```python
from build123d import *

# Parameters (mm, degrees)
F0_W      = 4.96
F0_H      = 15.83
F1_DEPTH  = 6.36
F2_R      = 2.45
F3_DEPTH  = 1.84
F4_R      = 2.45
F5_DEPTH  = 1.87
F6_R      = 2.45
F7_DEPTH  = 1.87
F9_D      = 3.14
F10_R     = 2.45
F11_DEPTH = 1.43
F12_R     = 2.45
F13_DEPTH = 1.43
F14_R     = 1.57
F15_DEPTH = 5.06
F16_R     = 1.57
F17_DEPTH = 1.43
F18_R     = 1.6
F19_DEPTH = 6.435
F20_R     = 1.7
F21_DEPTH = 1.41
F22_R     = 1.6
F23_DEPTH = 6.435
F24_R     = 1.7
F25_DEPTH = 1.41


with BuildPart() as f1:
    # F0 (on Front) → F1 (new body)
    with BuildSketch(Plane.XZ):
        with Locations((-27.94799, 11.446154)):
            Rectangle(F0_W, F0_H)
    extrude(amount=F1_DEPTH)

    # F2 (on face) → F3 (join)
    with BuildSketch(Plane.XZ.offset(6.36)):
        with Locations((-27.94799, 15.941154)):
            Circle(F2_R)
    extrude(amount=F3_DEPTH)

    # F4 (on face) → F5 (join)
    with BuildSketch(Plane.XY.offset(19.361154)):
        with Locations((-27.94799, -3.18)):
            Circle(F4_R)
    extrude(amount=F5_DEPTH)

    # F6 (on face) → F7 (join)
    with BuildSketch(Plane(origin=(0, 0, 3.531154), x_dir=(1, 0, 0), z_dir=(0, 0, -1))):
        with Locations((-27.94799, 3.18)):
            Circle(F6_R)
    extrude(amount=F7_DEPTH)

    # F9 (through all)
    with Locations(Plane(origin=(0, 0, 1.661154), x_dir=(1, 0, 0), z_dir=(0, 0, -1))):
        with Locations((-27.94799, 3.18)):
            Hole(F9_D / 2)

    # F10 (on face) → F11 (join)
    with BuildSketch(Plane.YZ.offset(-25.46799)):
        with Locations((-3.18, 15.941154)):
            Circle(F10_R)
    extrude(amount=F11_DEPTH)

    # F12 (on face) → F13 (join)
    with BuildSketch(Plane(origin=(-30.42799, 0, 0), x_dir=(0, -1, 0), z_dir=(-1, 0, 0))):
        with Locations((3.18, 15.941154)):
            Circle(F12_R)
    extrude(amount=F13_DEPTH)

    # F14 (on face) → F15 (join)
    with BuildSketch(Plane.XZ.offset(6.36)):
        with Locations((-27.94799, 6.951154)):
            Circle(F14_R)
    extrude(amount=F15_DEPTH)

    # F16 (on face) → F17 (join)
    with BuildSketch(Plane(origin=(0, 0, 0), x_dir=(-1, 0, 0), z_dir=(0, 1, 0))):
        with Locations((27.94799, 15.941154)):
            Circle(F16_R)
        with Locations((27.94799, 6.951154)):
            Circle(F16_R)
    extrude(amount=F17_DEPTH)

    # F18 (on face) → F19 (join)
    with BuildSketch(Plane(origin=(-31.85799, 0, 0), x_dir=(0, -1, 0), z_dir=(-1, 0, 0))):
        with Locations((3.18, 15.941154)):
            Circle(F18_R)
    extrude(amount=F19_DEPTH)

    # F20 (on face) → F21 (join)
    with BuildSketch(Plane(origin=(-38.29299, 0, 0), x_dir=(0, -1, 0), z_dir=(-1, 0, 0))):
        with Locations((3.18, 15.941154)):
            Circle(F20_R)
    extrude(amount=F21_DEPTH)

    # F22 (on face) → F23 (join)
    with BuildSketch(Plane.YZ.offset(-24.03799)):
        with Locations((-3.18, 15.941154)):
            Circle(F22_R)
    extrude(amount=F23_DEPTH)

    # F24 (on face) → F25 (join)
    with BuildSketch(Plane.YZ.offset(-17.60299)):
        with Locations((-3.18, 15.941154)):
            Circle(F24_R)
    extrude(amount=F25_DEPTH)


solid = f1.part
```
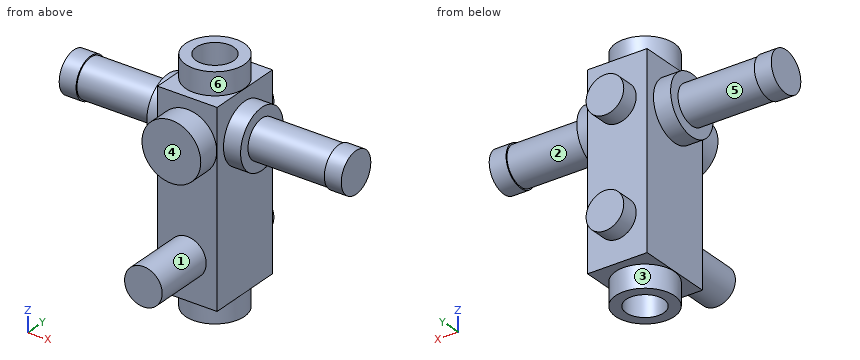
Geometry: final body of the model. Coordinates: model frame, mm. Face numbers are marked on the shaded views. A direction names the side the tool comes from. Round coordinates to 2 decimals unless told otherwise and drop trailing zeros. Write each loop counter-clockwise with the first axis right and the second up, starting at its lowest first coordinate (ties: lowest second). Pieces come first, ordered by that corner, then holes.
Item 1: Mould query, pull axis Z, two halves, no side actions, for the marked faces 1, 2 and 3. Classes: +Z half, -Z half, draft (parallel to the pull), parting line (faces both ways), or undercut.
Item 2: Set-up query: the marked faces 4, 5 and 6. Return all of +Z, -Z, +X, -X, +Y, -Y with unobstructed straight access to the full face (end or side cutting, diameter ignored); none if empty.
Item 3: Pin query (flat end, axial travel): P1, Ø1.5, axis at y = -8, z = 18, coming from the +X side; P2, Ø2, axis at x = -24, y = -1.5, coming from the +Z side; P3, Ø4, axis at x = -30.5, z = 15, coming from the -Y side. Return the tip coordinate at first contact, or that it passes through.
Item 4: Section query D-D (y = -10.25). Return loops of the section in (x, z).
Item 5: Section query A-A (z = 18.75). Return loops of the section in (x, y), plus the area to 3 significant figures.
Item 6: Material intervals for L1, parallel to X at y = -5.25, z = 8.5; L2, parallel to X at y = -4.5, z = 6.5; L3, parallel to Z at x = -35, y = -3.25, sorted ascending.
Item 7: Section query C-C (x = -20.75). Return loops of the section in (y, z), plus the area to 3 significant figures.
Completed:
1. face 1: undercut
1. face 2: parting line
1. face 3: draft
2. face 4: +Z, +X, -X, -Y
2. face 5: none
2. face 6: +Z
3. P1: stops at x = -25.88
3. P2: stops at z = 18.29
3. P3: stops at y = -8.2
4. outline: circle Ø3.14 at (-27.95, 6.95)
5. outline: (-30.43, -6.36) - (-25.47, -6.36) - (-25.47, 0) - (-30.43, 0) - close; hole circle Ø3.14 at (-27.95, -3.18)
5. area: 23.8 mm2
6. L1: x = -30.43 to -25.47
6. L2: x = -30.43 to -28.8, -27.1 to -25.47
6. L3: z = 14.34 to 17.54
7. outline: circle Ø3.2 at (-3.18, 15.94)
7. area: 8.04 mm2
